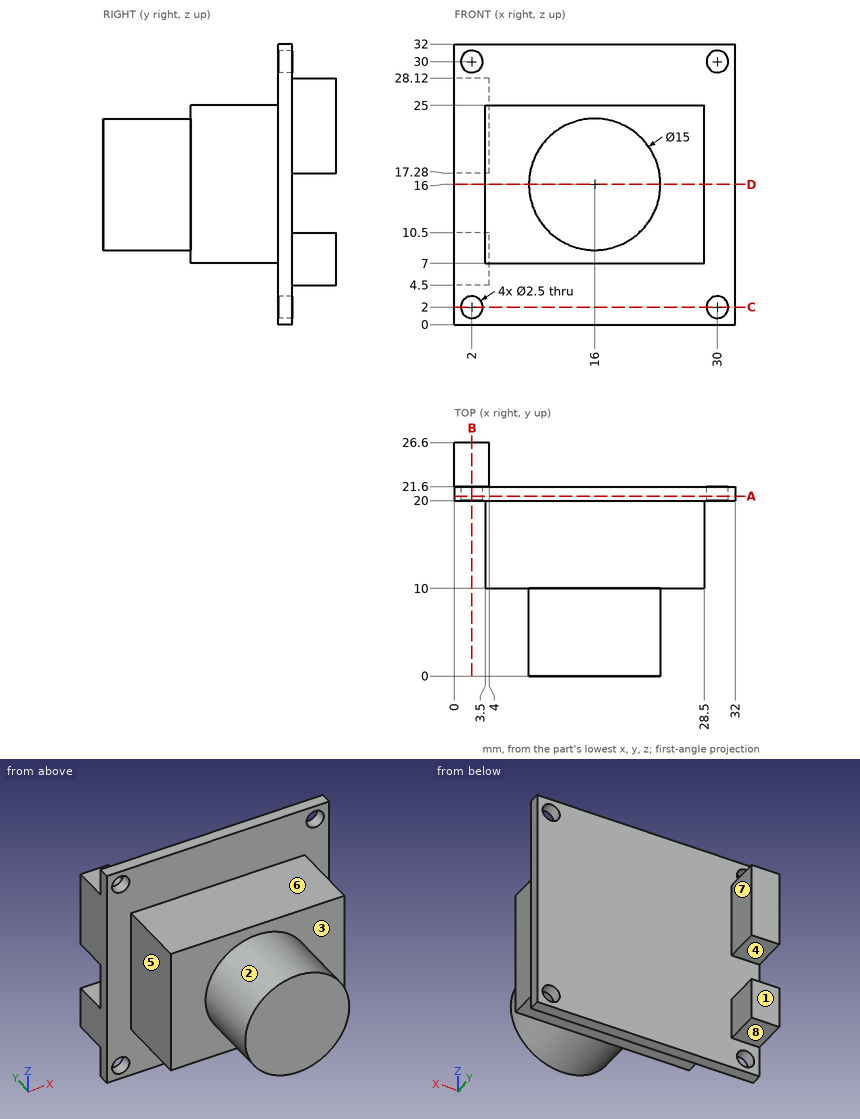
Job drawing, mm, ordinate dimensions from the low corner. One solid piece. A direction names the side the tool comes from. Give positions to 0.01 mm unless a question says otherwise; leave off trailing zeros. Loops run counter-clockwise (first coordinate to the right, second up) from the corner with the lowest first, then second, coordinate; pieces in that order, holes last.
Item 1: Slice it at A-A, the plane y = 20.5. List the corners of the cut face in (x, z).
Answers follow:
outline: (0, 0) - (32, 0) - (32, 32) - (0, 32) - close; hole circle Ø2.5 at (2, 2); hole circle Ø2.5 at (2, 30); hole circle Ø2.5 at (30, 2); hole circle Ø2.5 at (30, 30)
Item 2: Pull direction Y, two halves, no side cores. Call the marked faces 1, 2 and 3: released by +Y, released by -Y, zero draft, split by the parting line, or undercut.
Answers follow:
face 1: released by +Y
face 2: zero draft
face 3: released by -Y
Item 3: Slice it at C-C, the plane z = 2. List the corners of the cut face in (x, y), and give its area (3 significant figures).
Answers follow:
outline: (0, 20) - (0.75, 20) - (0.75, 21.6) - (0, 21.6) - close; (3.25, 20) - (28.75, 20) - (28.75, 21.6) - (3.25, 21.6) - close; (31.25, 20) - (32, 20) - (32, 21.6) - (31.25, 21.6) - close
area: 43.2 mm2
Item 4: Flat gauge pins, fed straight in: pin 1 (3 mm diameter, centred on x = 30, z = 2, fed in from -Y); pin 2 (8 mm diameter, centred on x = 8, z = 11.5, fed in from +Y); pin 3 (3 mm diameter, centred on y = 15.5, z = 13, fed in from +X); pin 4 (4 mm diameter, centred on x = 12.5, y = 22, fed in from -Z). Where does each tip first touch, or does it go through?
Answers follow:
pin 1: stops at y = 20
pin 2: stops at y = 21.6
pin 3: stops at x = 28.5
pin 4: stops at z = 0
Item 5: Slice it at B-B, the plane x = 2. List the corners of the cut face in (y, z), and give its area (3 significant figures).
Answers follow:
outline: (20, 0) - (21.6, 0) - (21.6, 0.75) - (20, 0.75) - close; (20, 3.25) - (21.6, 3.25) - (21.6, 4.5) - (26.6, 4.5) - (26.6, 10.5) - (21.6, 10.5) - (21.6, 17.28) - (26.6, 17.28) - (26.6, 28.12) - (21.6, 28.12) - (21.6, 28.75) - (20, 28.75) - close; (20, 31.25) - (21.6, 31.25) - (21.6, 32) - (20, 32) - close
area: 127 mm2
Item 6: Slice it at D-D, the plane z = 16. List the corners of the cut face in (x, y), and give its area (3 significant figures).
Answers follow:
outline: (0, 20) - (3.5, 20) - (3.5, 10) - (8.5, 10) - (8.5, 0) - (23.5, 0) - (23.5, 10) - (28.5, 10) - (28.5, 20) - (32, 20) - (32, 21.6) - (0, 21.6) - close
area: 451 mm2
Item 7: Which spindle directions (+Z, -Z, +X, -X, +Y, -Y) get a long thin tool onto all of the face, cutting with end or side? Do the marked faces 4, 5, 6, 7 and 8. Say none if no direction does.
Answers follow:
face 4: +X, -X, +Y
face 5: +Z, -Z, -X, -Y
face 6: +Z, +X, -X, -Y
face 7: +Z, -Z, +X, +Y
face 8: -Z, +X, -X, +Y
Item 8: Drill centre lines: line 1 (Z direction, x = 30, y = 20.4); line 2 (Y direction, x = 14, z = 25.5); line 3 (X direction, y = 23.5, z = 8.5). Where is each one in solid material? Low to high.
Answers follow:
line 1: z = 0 to 0.75, 3.25 to 28.75, 31.25 to 32
line 2: y = 20 to 21.6
line 3: x = 0 to 4
